Autodesk Inventor part; units mm, degrees
ref_plane "YZ Plane" through (0, 0, 0) normal (1, 0, 0) x (0, 1, 0)
ref_plane "XZ Plane" through (0, 0, 0) normal (0, 1, 0) x (-1, 0, 0)
ref_plane "XY Plane" through (0, 0, 0) normal (0, 0, 1) x (1, 0, 0)
sketch "Sketch1" plane through (0, 0, 0) normal (0, 1, 0) x (-1, 0, 0)
  line L0 (6.5, -8) -> (-6.5, -8)
  line L1 (-6.5, -8) -> (-6.5, 8)
  line L2 (-6.5, 8) -> (6.5, 8)
  line L3 (6.5, 8) -> (6.5, -8)
  line L4 (6.5, -8) -> (-6.5, 8) construction
  line L5 (-6.5, -8) -> (6.5, 8) construction
  line L6 (5.5, -7) -> (-5.5, -7)
  line L7 (-5.5, -7) -> (-5.5, 7)
  line L8 (-5.5, 7) -> (5.5, 7)
  line L9 (5.5, 7) -> (5.5, -7)
  point P0 (0, 0)
  dimension "d0" = 13
  dimension "d1" = 16
  dimension "d2" = 1
extrude "Extrusion1" add sketch "Sketch1" along normal blind 1.5
fillet "Fillet1" radius 2 4 edges at (-5.5, 0.75, -7) (-5.5, 0.75, 7) (5.5, 0.75, 7) (5.5, 0.75, -7)
properties part number "cellSTORM_chip_chamber"
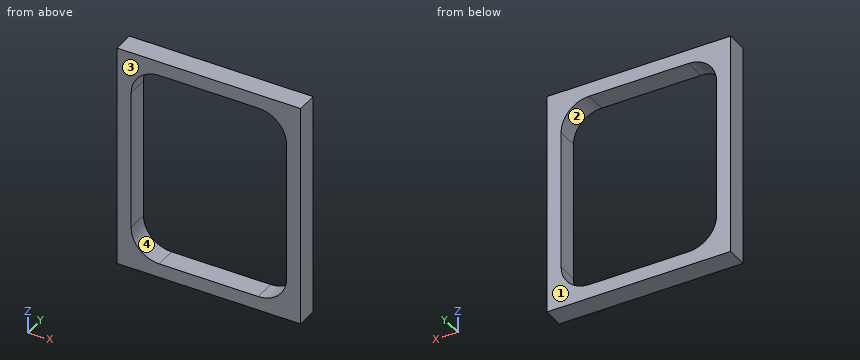
CAD build for the part. Positions are in the model's coordinates, mm. Face numbers are marked on the shaded views. A direction names the side the tool comes from. Give positions to 0.01 mm unless a question says otherwise; leave off trailing zeros. Order: outer loops, then holes, each group sorted by start corner. A loop starts at its lowest first (then second) coordinate and runs counter-clockwise, first axis right, second up. Notation, with made-up numbers: (-40, 43.25) -> (4, 43.25) arc R12 cw to (4, 63.25) -> close; hole circle Ø10 at (-29.75, -4.5). An arc over 180 degrees is marked (long way). Return JSON: item names as keys, results as strings.
Q1. Saw through at B-B (y = 1.3). Write the cut outline in (x, z), then the cut area to 3 significant figures.
Working result:
{"outline": "(-6.5, -8) -> (6.5, -8) -> (6.5, 8) -> (-6.5, 8) -> close; hole (-5.5, -5) arc R2 ccw to (-3.5, -7) -> (3.5, -7) arc R2 ccw to (5.5, -5) -> (5.5, 5) arc R2 ccw to (3.5, 7) -> (-3.5, 7) arc R2 ccw to (-5.5, 5) -> close", "area": "57.4 mm²"}
Q2. Saw through at A-A (z = -0.5). Write the cut outline in (x, y).
Working result:
{"outline": "(-6.5, 0) -> (-5.5, 0) -> (-5.5, 1.5) -> (-6.5, 1.5) -> close; (5.5, 0) -> (6.5, 0) -> (6.5, 1.5) -> (5.5, 1.5) -> close"}
Q3. Saw through at C-C (x = -2.5). Write the cut outline in (y, z), then the cut area to 3 significant figures.
Working result:
{"outline": "(0, -8) -> (1.5, -8) -> (1.5, -7) -> (0, -7) -> close; (0, 7) -> (1.5, 7) -> (1.5, 8) -> (0, 8) -> close", "area": "3.00 mm²"}
Q4. Drill centre lines: line 1 (Z direction, x = 1.5, y = 0.95); line 2 (X direction, y = 0.25, z = -1.5); line 3 (Z direction, x = 4.5, y = 1.45). Where is each one in solid material? Low to high.
Working result:
{"line 1": "-8 to -7, 7 to 8", "line 2": "-6.5 to -5.5, 5.5 to 6.5", "line 3": "-8 to -6.73, 6.73 to 8"}
Q5. Which spindle directions (+Z, -Z, +X, -X, +Y, -Y) get a long thin tool onto all of the face, cutting with end or side? Do the marked faces 3 and 4. Say none if no direction does.
Working result:
{"face 3": "+Z, -Z, +X, -X, -Y", "face 4": "+Y, -Y"}
Q6. Mould opens along Z. For the marked faces 1 and 2 say: pulls with the +Z half, pulls with the -Z half, needs draft (parallel to the pull), parting line crosses it, or undercut.
Working result:
{"face 1": "needs draft", "face 2": "undercut"}
